Drawing for the job (mm, zero at the part's lowest x, y, z). A direction names the side the tool comes from. Coordinates: 2 decimals unless noted, no trailing zeros. Write each loop counter-clockwise with the first axis right and the second up, starting at its lowest first coordinate (ties: lowest second). Pieces come first, ordered by that corner, then holes. Notation, with made-up numbers: M 10.25,-17.5 L 54.25,-17.5 A28 cw 54.25,15.5 Z; hole C 75,-28.75 d7. An arc over 180 degrees is marked long. Use a Markdown table: item, result. Add a question column.
Q1. Tool access for the marked faces 1 and 2: list every direction of +Z, -Z, +X, -X, +Y, -Y with a clear straight run to the whole face (end or side of a thin tool).
Q2. Wall check: L1, parallel to X at y = 10.5, z = 6.25; L2, parallel to Z at x = 5, y = 43; L3, parallel to Z at x = 4.25, y = 45. Give the ranges that are in metal, low to high. Write a range as from..to.
Q3. Slice it at A-A on y = 11.5. Write the cut outline in (x, z).
Q4. Pin check, flat tips, straight feed: pin 1 Ø3 at (x, y) = (7, 41) entering from -Z; pin 2 Ø1 at (x, z) = (6.5, 5) entering from -Y; pin 3 Ø2 at (x, y) = (7, 30.5) entering from +Z. Stop position of each tip, or through.
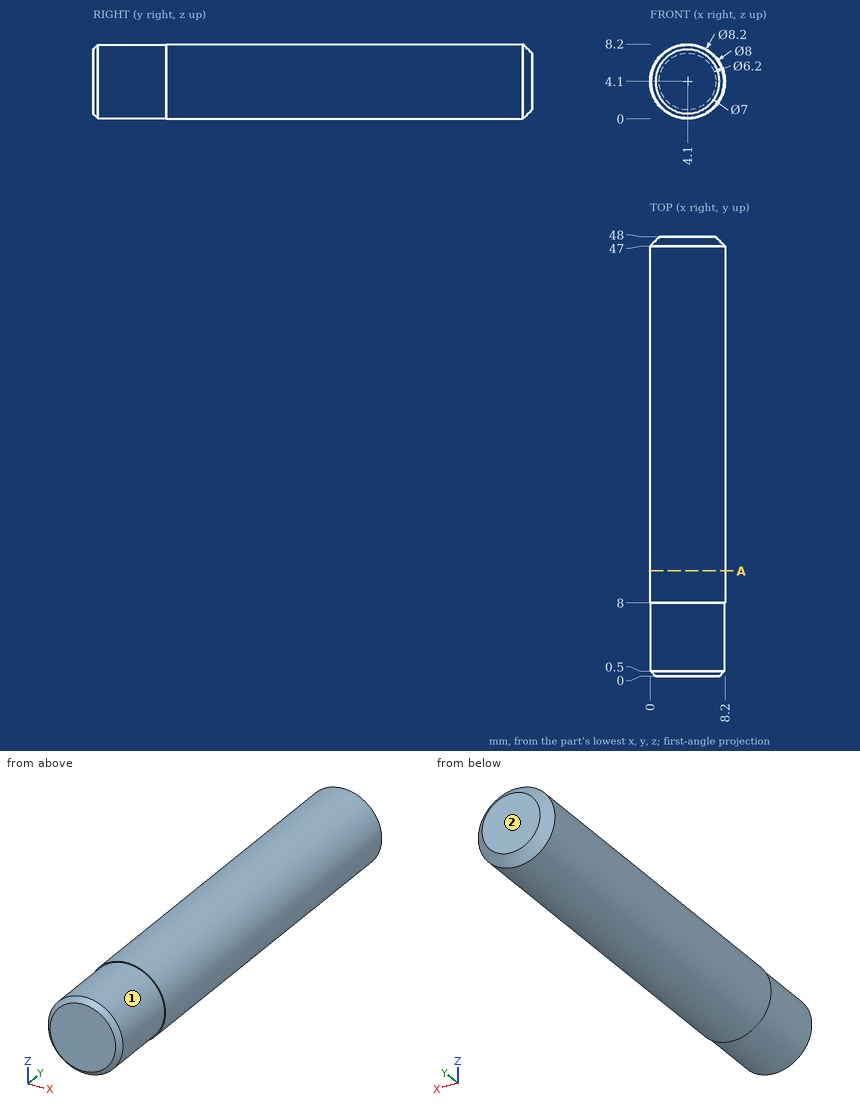
Recorded:
| question | item | result |
|---|---|---|
| 1 | face 1 | -Y |
| 1 | face 2 | +Z, -Z, +X, -X, +Y |
| 2 | L1 | 0.61..7.59 |
| 2 | L2 | 0.1..8.1 |
| 2 | L3 | 0..8.2 |
| 3 | outline | C 4.1,4.1 d8.2 |
| 4 | pin 1 | z = 0.25 |
| 4 | pin 2 | y = 0 |
| 4 | pin 3 | z = 7.73 |
